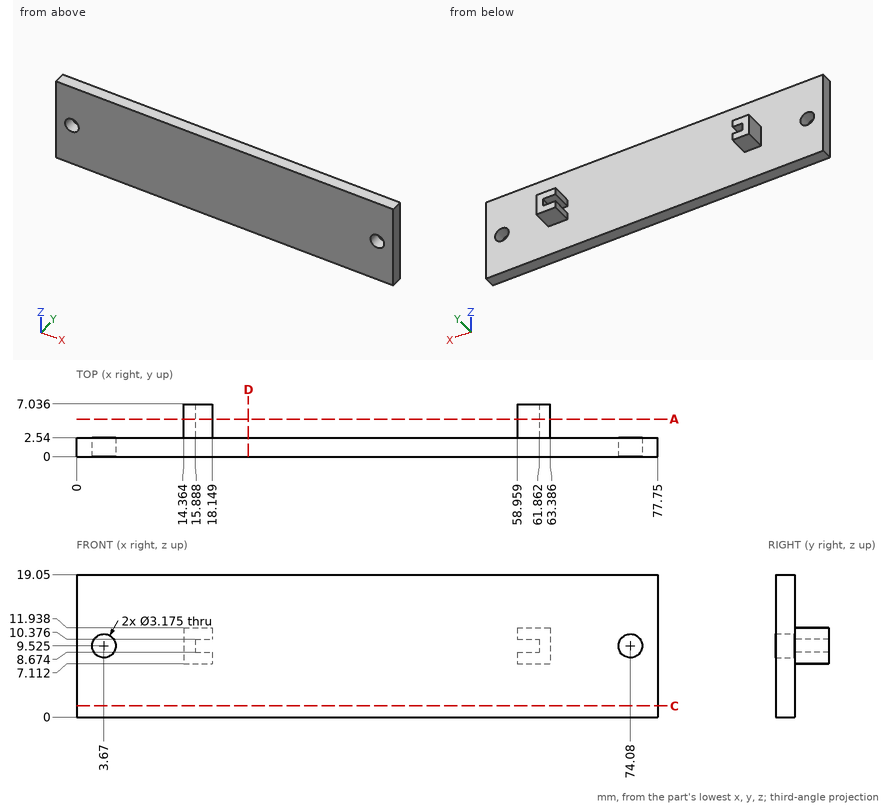
Input: dimensioned drawing with shaded views. Units: mm. Origin: part minimum x, y, z. Coordinates: 2 decimals unless noted, no trailing zeros. Order: outer loops, then holes, each group sorted by start corner. A loop starts at its lowest first (then second) coordinate and runs counter-clockwise, first axis right, second up.
(1) Section query C-C (z = 1.5). Return the cut outline in (x, y).
(2) Material intervals for probe 1 along X at (y, z) = (2.25, 9.75); probe 2 along X at (y, z) = (2, 9.25); probe 3 along X at (y, z) = (5.5, 11.5), sorted ascending.
(3) First-contact query: pin 1 (3 mm diameter, centred on x = 11, z = 5, fed in from +Y); pin 2 (1.2 mm diameter, centred on y = 4, z = 8, fed in from +X); pin 3 (3 mm diameter, centred on x = 60, y = 5, fed in from -Z). Flat tips, straight axial feed; report the tip coordinate or a pass-through.
(4) Section query A-A (y = 5). Return the cut outline in (x, z).
(5) Section query D-D (x = 23). Return the cut outline in (y, z), plus the area to 3 significant figures.
Solution:
1. outline: (0, 0) - (77.75, 0) - (77.75, 2.54) - (0, 2.54) - close
2. probe 1: x = 0 to 2.1, 5.24 to 72.51, 75.65 to 77.75
2. probe 2: x = 0 to 2.11, 5.23 to 72.52, 75.64 to 77.75
2. probe 3: x = 14.36 to 18.15, 58.96 to 63.39
3. pin 1: stops at y = 2.54
3. pin 2: stops at x = 63.39
3. pin 3: stops at z = 7.11
4. outline: (14.36, 7.11) - (18.15, 7.11) - (18.15, 8.67) - (15.89, 8.67) - (15.89, 10.38) - (18.15, 10.38) - (18.15, 11.94) - (14.36, 11.94) - close; (58.96, 7.11) - (63.39, 7.11) - (63.39, 11.94) - (58.96, 11.94) - (58.96, 10.38) - (61.86, 10.38) - (61.86, 8.67) - (58.96, 8.67) - close
5. outline: (0, 0) - (2.54, 0) - (2.54, 19.05) - (0, 19.05) - close
5. area: 48.4 mm2
